Input: dimensioned drawing with shaded views. Units: mm. Origin: part minimum x, y, z. A direction names the side the tool comes from. Give positions to 0.01 mm unless a question says otherwise; leave off trailing zeros. Loops run counter-clockwise (first coordinate to the right, second up) from the corner with the lowest first, then second, coordinate; pieces in that order, holes last. Notation, with made-up numbers: M 30.5,-6.75 L 78.5,-6.75 A22 ccw 78.5,27.25 Z; hole C 83.5,56.25 d5. An arc over 180 degrees is marked long. Answer in a Markdown table with one row per item.
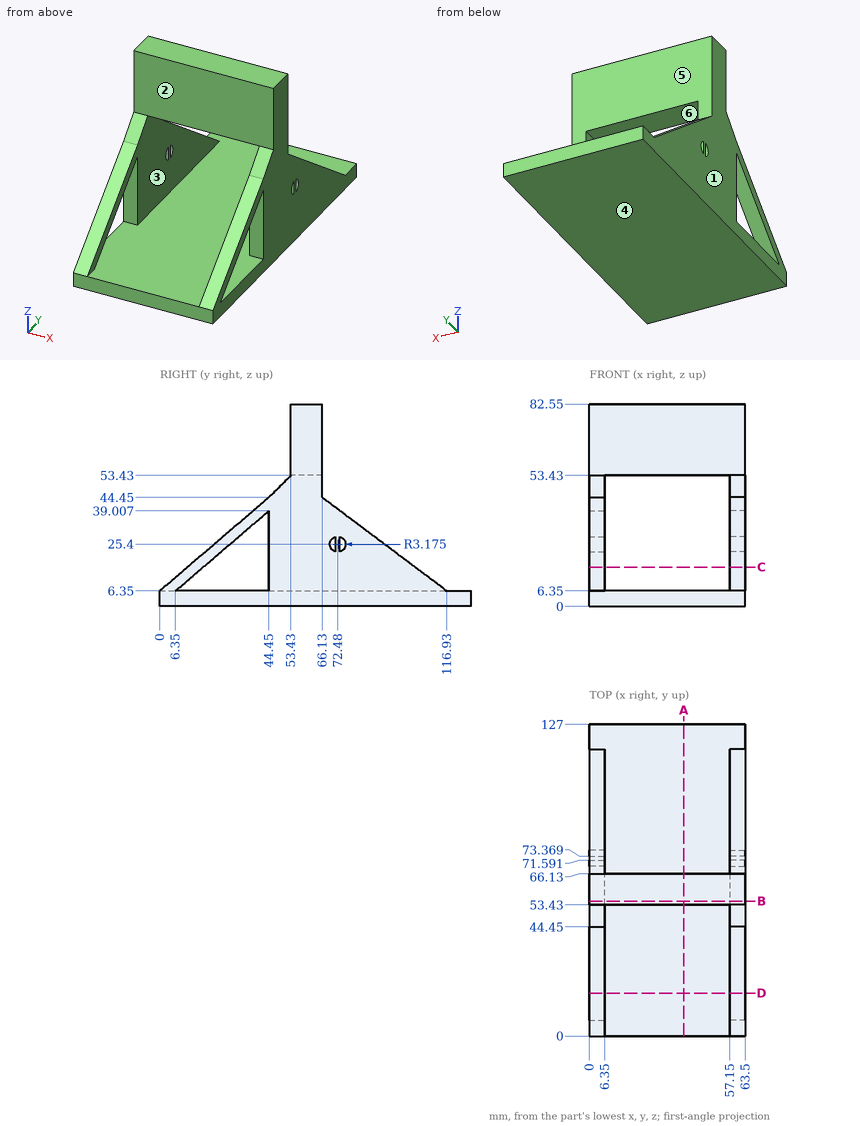
Q1. Section query B-B (y = 55). Output: boundary loops of the cut face in (x, z).
Values follow:
| item | result |
|---|---|
| outline | M 0,0 L 63.5,0 L 63.5,82.55 L 0,82.55 Z; hole M 6.35,6.35 L 57.15,6.35 L 57.15,53.43 L 6.35,53.43 Z |
Q2. Section query D-D (y = 17.5). Output: boundary loops of the cut face in (x, z).
Values follow:
| item | result |
|---|---|
| outline | M 0,0 L 63.5,0 L 63.5,6.35 L 0,6.35 Z; M 0,15.91 L 6.35,15.91 L 6.35,21.35 L 0,21.35 Z; M 57.15,15.91 L 63.5,15.91 L 63.5,21.35 L 57.15,21.35 Z |
Q3. Ray query, probe 1 along X at (y, z) = (33.5, 34.5); probe 2 along Z at (x, y) = (51, 8.5); probe 3 along Z at (x, y) = (51.5, 66). Return the intervals inside material, ascending. Write a range as from..to.
Values follow:
| item | result |
|---|---|
| probe 1 | 0..6.35, 57.15..63.5 |
| probe 2 | 0..6.35 |
| probe 3 | 0..6.35, 53.43..82.55 |
Q4. Reachability of the marked faces 1, 2 and 3 from +Z, -Z, +X, -X, +Y, -Y: full face, straight path, thin tool, end or side. Return the list, or none.
Values follow:
| item | result |
|---|---|
| face 1 | +Z, -Z, -X, +Y, -Y |
| face 2 | +Z, +X, -X, -Y |
| face 3 | +Y, -Y |
Q5. Contact query for flat-ended pins moving along their axis: pin 1 Ø1.8 at (x, z) = (2.5, 26.5) entering from -Y; pin 2 Ø7 at (x, z) = (61.5, 30.5) entering from -Y; pin 3 Ø7 at (x, z) = (2.5, 23) entering from -Y. Output: stop coordinate, or through.
Values follow:
| item | result |
|---|---|
| pin 1 | y = 22.46 |
| pin 2 | y = 24.09 |
| pin 3 | y = 15.34 |
Q6. Section query A-A (x = 38.5). Output: boundary loops of the cut face in (y, z).
Values follow:
| item | result |
|---|---|
| outline | M 0,0 L 127,0 L 127,6.35 L 0,6.35 Z; M 53.43,53.43 L 66.13,53.43 L 66.13,82.55 L 53.43,82.55 Z |
Q7. Mould query, pull axis Z, two halves, no side actions, for the marked faces 4, 5 and 6. Classes: +Z half, -Z half, draft (parallel to the pull), parting line (faces both ways), or undercut.
Values follow:
| item | result |
|---|---|
| face 4 | -Z half |
| face 5 | draft |
| face 6 | undercut |
Q8. Section query C-C (z = 16). Output: boundary loops of the cut face in (x, y), plus the area to 3 significant figures.
Values follow:
| item | result |
|---|---|
| outline | M 0,11.26 L 6.35,11.26 L 6.35,17.61 L 0,17.61 Z; M 0,44.45 L 6.35,44.45 L 6.35,104.06 L 0,104.06 Z; M 57.15,11.26 L 63.5,11.26 L 63.5,17.61 L 57.15,17.61 Z; M 57.15,44.45 L 63.5,44.45 L 63.5,104.06 L 57.15,104.06 Z |
| area | 838 mm^2 |
